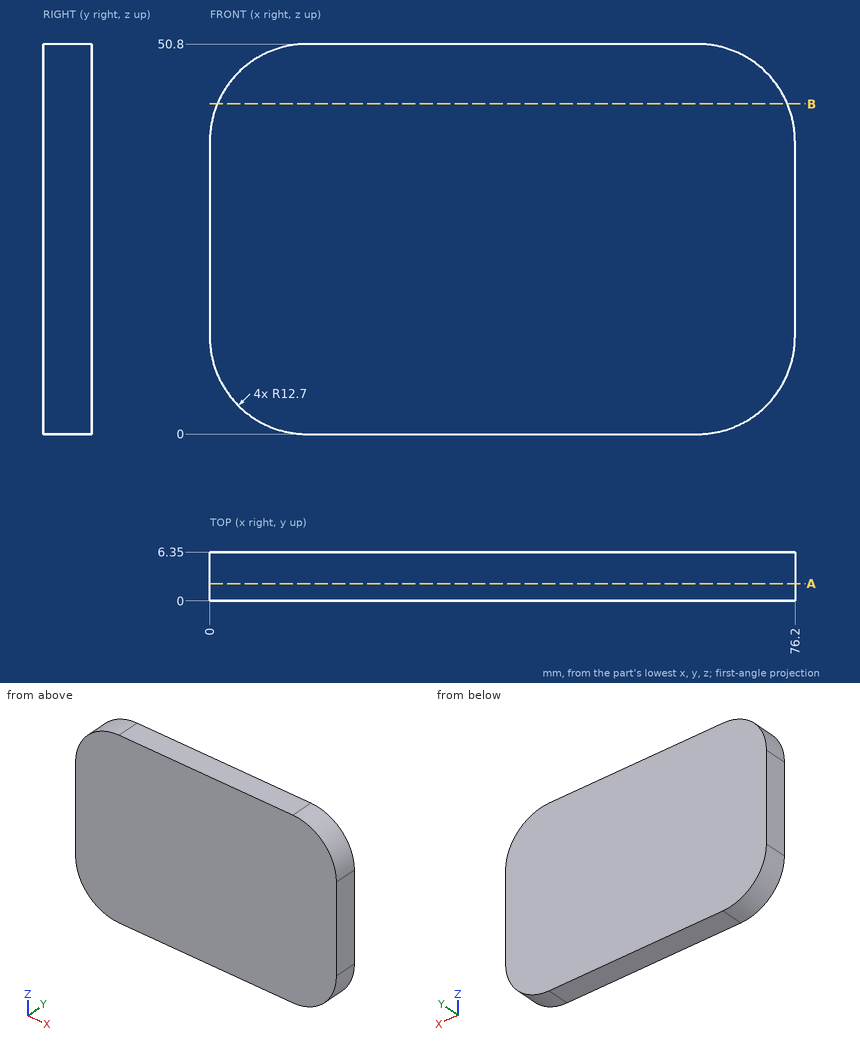
Here's the drawing with two shaded views (mm, measured from the low corner). I have some questions. Give positions to 0.01 mm unless a question says otherwise; leave off trailing zeros. Write each loop counter-clockwise with the first axis right and the second up, starting at its lowest first coordinate (ties: lowest second). Pieces come first, ordered by that corner, then holes. Notation, with made-up numbers: (50.25, 46) - (61.25, 46) arc R28 cw to (61.25, 69) - close; hole circle Ø5 at (-29.5, 83.5). An arc over 180 degrees is marked (long way). Write item = value, one per line. Start each with the question number.
1. Imagine slicing it at A-A (y = 2.25). Please give me the cut outline in (x, z).
2. Imagine slicing it at B-B (z = 43). Please give me the cut outline in (x, y), and give its area (3 significant figures).
3. Please list where these lines run through material, in increasing order: line 1 (X direction, y = 2.75, z = 10.5); line 2 (Z direction, x = 67.5, y = 3); line 3 (X direction, y = 5, z = 12.5).
4. For pin 1 (1 mm diameter, centred on y = 3.5, z = 5, fed in from +X); pin 2 (1.5 mm diameter, centred on x = 11.5, y = 5, fed in from -Z), each with a flat end and sliding along its axis, tell me the tip position at first contact or that it passes through.
Worked answers:
q1.outline = (0, 12.7) arc R12.7 ccw to (12.7, 0) - (63.5, 0) arc R12.7 ccw to (76.2, 12.7) - (76.2, 38.1) arc R12.7 ccw to (63.5, 50.8) - (12.7, 50.8) arc R12.7 ccw to (0, 38.1) - close
q2.outline = (0.98, 0) - (75.22, 0) - (75.22, 6.35) - (0.98, 6.35) - close
q2.area = 471 mm2
q3.line_1 = 0.19 to 76.01
q3.line_2 = 0.65 to 50.15
q3.line_3 = 0 to 76.2
q4.pin_1 = 73.96
q4.pin_2 = 0.01
